Part model, mm, in its own coordinate system. Face numbers are marked on the shaded views. A direction names the side the tool comes from. Give positions to 0.01 mm unless a question says otherwise; leave off trailing zeros. Write each loop counter-clockwise with the first axis right and the second up, starting at its lowest first coordinate (ties: lowest second). Pieces come first, ordered by that corner, then holes. Notation, with made-up numbers: (-28, 86.25) - (25, 86.25) arc R5 ccw to (25, 93.25) - close; hole circle Ø11 at (-12.75, 51.25). An arc over 180 degrees is marked (long way). Answer in a Markdown table with one row per item. Add a question column.
1. Pull direction Y, two halves, no side cores. Call the marked faces 3, 4 and 5: released by +Y, released by -Y, zero draft, split by the parting line, or undercut.
2. Band-saw the part on A-A on z = 15.5. Write the cut outline in (x, y), plus the area to 3 significant figures.
3. Band-saw the part on D-D on y = -27. Write the cut outline in (x, z), plus the area to 3 significant figures.
4. Probe line 1 along Z through (x, y) = (22.5, -50); line 2 along X through (y, z) = (-50, 32.5); line 3 along Y through (x, z) = (19.5, 4.5). List the from-to ranges inside material, lowest first.
5. Band-saw the part on C-C on y = -35. Write the cut outline in (x, z), plus the area to 3 significant figures.
6. Which spindle directions (+Z, -Z, +X, -X, +Y, -Y) get a long thin tool onto all of the face, cutting with end or side? Do the marked faces 1 and 2. Say none if no direction does.
7. Drop flat-ended pins along their axis: pin 1 Ø19 at (y, z) = (-28.575, 28.575) entering from +X; pin 2 Ø10 at (x, y) = (34.5, -22) entering from +Z. Give the stop position or say it passes through.
8. Band-saw the part on B-B on x = 21. Write the cut outline in (y, z), plus the area to 3 significant figures.
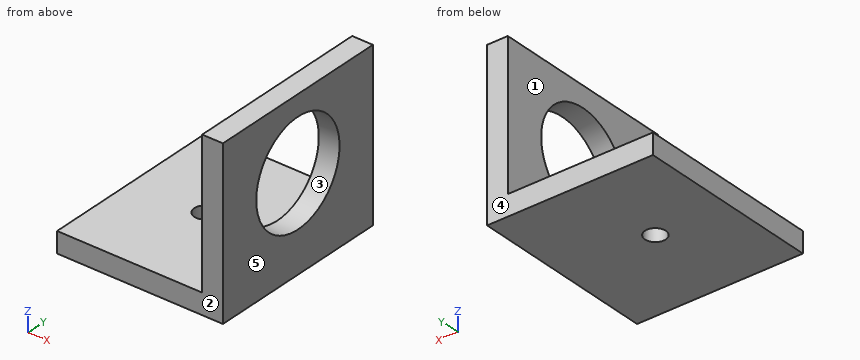
```python
from build123d import *

# Parameters (mm, degrees)
F1_DEPTH = 57.15
F2_R     = 15.875
F3_DEPTH = 6.351
F4_R     = 3.175
F5_DEPTH = 6.351


with BuildPart() as f1:
    # F0 (on Front) → F1 (new body)
    with BuildSketch(Plane.XZ):
        Polygon((0, 6.35), (0, 0), (50.8, 0), (50.8, 50.8), (44.45, 50.8), (44.45, 6.35), align=None)
    extrude(amount=F1_DEPTH)

    # F2 (on face) → F3 (cut, through all)
    with BuildSketch(Plane(origin=(44.45, 0, 0), x_dir=(0, -1, 0), z_dir=(-1, 0, 0))):
        with Locations((28.575, 28.575)):
            Circle(F2_R)
    extrude(amount=-F3_DEPTH, mode=Mode.SUBTRACT)

    # F4 (on face) → F5 (cut, through all)
    with BuildSketch(Plane.XY.offset(6.35)):
        with Locations((22.225, -28.575)):
            Circle(F4_R)
    extrude(amount=-F5_DEPTH, mode=Mode.SUBTRACT)


solid = f1.part
```
Values:
| question | item | result |
|---|---|---|
| 1 | face 3 | undercut |
| 1 | face 4 | released by +Y |
| 1 | face 5 | zero draft |
| 2 | outline | (44.45, -57.15) - (50.8, -57.15) - (50.8, -37.58) - (44.45, -37.58) - close; (44.45, -19.57) - (50.8, -19.57) - (50.8, 0) - (44.45, 0) - close |
| 2 | area | 249 mm² |
| 3 | outline | (0, 0) - (19.47, 0) - (19.47, 6.35) - (0, 6.35) - close; (24.98, 0) - (50.8, 0) - (50.8, 12.78) - (44.45, 12.78) - (44.45, 6.35) - (24.98, 6.35) - close; (44.45, 44.37) - (50.8, 44.37) - (50.8, 50.8) - (44.45, 50.8) - close |
| 3 | area | 369 mm² |
| 4 | line 1 | z = 0 to 6.35 |
| 4 | line 2 | x = 44.45 to 50.8 |
| 4 | line 3 | y = -57.15 to -30.2, -26.95 to 0 |
| 5 | outline | (0, 0) - (50.8, 0) - (50.8, 14.06) - (44.45, 14.06) - (44.45, 6.35) - (0, 6.35) - close; (44.45, 43.09) - (50.8, 43.09) - (50.8, 50.8) - (44.45, 50.8) - close |
| 5 | area | 420 mm² |
| 6 | face 1 | +Z, -X, +Y, -Y |
| 6 | face 2 | +Z, -Z, +X, -X, -Y |
| 7 | pin 1 | passes through |
| 7 | pin 2 | stops at z = 6.35 |
| 8 | outline | (-57.15, 0) - (-31.5, 0) - (-31.5, 6.35) - (-57.15, 6.35) - close; (-25.65, 0) - (0, 0) - (0, 6.35) - (-25.65, 6.35) - close |
| 8 | area | 326 mm² |
